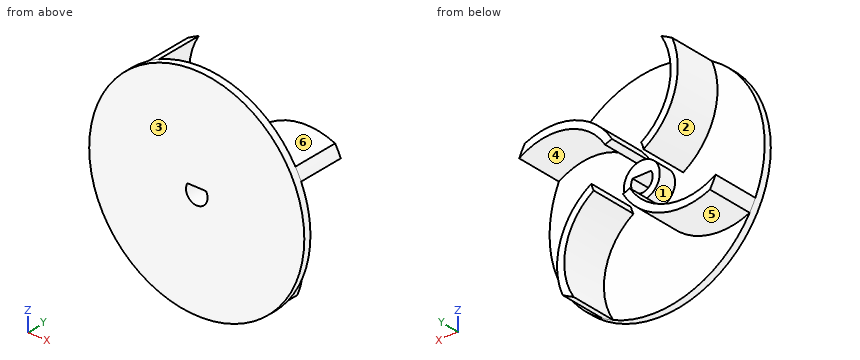
from build123d import *

# Parameters (mm, degrees)
SKETCH1_R           = 30
BOSS_EXTRUDE1_DEPTH = 2
SKETCH2_R           = 5
BOSS_EXTRUDE2_DEPTH = 7
BOSS_EXTRUDE3_DEPTH = 13
CUT_EXTRUDE1_DEPTH  = 16
CIRPATTERN2_COUNT   = 4


with BuildPart() as part:
    # Sketch1 → Boss-Extrude1 (new body)
    with BuildSketch(Plane(origin=(0, 0, 0), x_dir=(1, 0, 0), z_dir=(0, 1, 0))):
        Circle(SKETCH1_R)
    extrude(amount=BOSS_EXTRUDE1_DEPTH)

    # Sketch2 → Boss-Extrude2 (add)
    with BuildSketch(Plane(origin=(0, 0, 0), x_dir=(1, 0, 0), z_dir=(0, 1, 0))):
        Circle(SKETCH2_R)
    extrude(amount=BOSS_EXTRUDE2_DEPTH)

    # Sketch3 → Boss-Extrude3 (add)
    with BuildSketch(Plane(origin=(0, 2, 0), x_dir=(1, 0, 0), z_dir=(0, 1, 0))):
        with BuildLine():
            ThreePointArc((-1.505806951, 7.292266896), (-12.151790035, 15.86929072), (-25.810761164, 15.290670625))
            ThreePointArc((-25.810761164, 15.290670625), (-26.649690738, 13.776573724), (-27.399897799, 12.216611666))
            ThreePointArc((-27.399897799, 12.216611666), (-14.251932533, 14.383859932), (-3.429686075, 6.60922571))
            ThreePointArc((-3.429686075, 6.60922571), (-2.491266579, 7.016993793), (-1.505806951, 7.292266896))
        make_face()
    boss_extrude3 = extrude(amount=BOSS_EXTRUDE3_DEPTH)

    # Sketch4 → Cut-Extrude1 (cut, through all)
    with BuildSketch(Plane(origin=(0, 0, 0), x_dir=(1, 0, 0), z_dir=(0, 1, 0))):
        with BuildLine():
            Line((-2.598076211, -1.5), (2.598076211, -1.5))
            ThreePointArc((2.598076211, -1.5), (0, 3), (-2.598076211, -1.5))
        make_face()
    extrude(amount=CUT_EXTRUDE1_DEPTH, mode=Mode.SUBTRACT)

    # CirPattern2: Boss-Extrude3 ×4 about axis
    cirpattern2_axis = Axis((0, 0, 0), (0, 1, 0))
    for i in range(1, CIRPATTERN2_COUNT):
        add(boss_extrude3.rotate(cirpattern2_axis, i * 360 / CIRPATTERN2_COUNT))


solid = part.part
Here's how the part is built. I have some questions about the finished solid (model axes, mm). Face numbers are marked on the shaded views. A direction names the side the tool comes from. Round coordinates to 2 decimals unless told otherwise and drop trailing zeros. Write each loop counter-clockwise with the first axis right and the second up, starting at its lowest first coordinate (ties: lowest second). Pieces come first, ordered by that corner, then holes.
1. Suppose I cut it at B-B (z = 0). List the corners of the cut face in (x, y) for me.
2. I need wall thicknesses on L1, parallel to Z at x = 0, y = 4.5; L2, parallel to X at y = 3, z = -2.5; L3, parallel to X at y = 2.25, z = 0. Which ranges of each line are inside material? Lowest first, please.
3. Will these pins go through, and if not, where does the flat tip stop? pin 1 Ø5 at (x, z) = (-1, 1) entering from +Y; pin 2 Ø6 at (x, z) = (4.5, -17) entering from +Y; pin 3 Ø5.5 at (x, y) = (-0.5, 2) entering from -Z; pin 4 Ø2 at (y, z) = (8.5, 3.5) entering from +X.
4. Suppose I cut it at A-A (y = 4.5). List the corners of the cut face in (x, z) for me, and give its area (3 significant figures).
5. Suppose I cut it at D-D (y = 13.25). List the corners of the cut face in (x, z) for me.
6. For the marked faces 4, 5 and 6, which set-ups out of +Z, -Z, +X, -X, +Y, -Y let a thin tool reach every point of the face, with its end or its side?
7. Suppose I cut it at C-C (x = 0). List the corners of the cut face in (y, z) for me.
8. If we mould it in two halves opening along X, with no side actions, what happens to the marked faces 1, 2 and 3? For each: released by +X, released by -X, zero draft, split by the parting line, or undercut.
Answer sheet:
1. outline: (-30, 0) - (-3, 0) - (-3, 7) - (-5, 7) - (-5, 2) - (-30, 2) - close; (3, 0) - (30, 0) - (30, 2) - (5, 2) - (5, 7) - (3, 7) - close
2. L1: z = -5 to -3, 1.5 to 5
2. L2: x = -4.33 to -1.66, 1.66 to 4.33, 7.01 to 8.81
2. L3: x = -5 to -3, 3 to 5
3. pin 1: stops at y = 7
3. pin 2: stops at y = 2
3. pin 3: stops at z = -30
3. pin 4: stops at x = -6.61
4. outline: (-27.4, -12.22) arc R30 ccw to (-25.81, -15.29) arc R19.39 ccw to (-1.51, -7.29) arc R7.45 cw to (-3.43, -6.61) arc R17.39 cw to start; (-15.29, 25.81) arc R19.39 ccw to (-7.29, 1.51) arc R7.45 cw to (-6.61, 3.43) arc R17.39 cw to (-12.22, 27.4) arc R30 ccw to start; circle Ø10 at (0, 0); (1.51, 7.29) arc R7.45 cw to (3.43, 6.61) arc R17.39 cw to (27.4, 12.22) arc R30 ccw to (25.81, 15.29) arc R19.39 ccw to start; (6.61, -3.43) arc R17.39 cw to (12.22, -27.4) arc R30 ccw to (15.29, -25.81) arc R19.39 ccw to (7.29, -1.51) arc R7.45 cw to start; hole (-2.6, 1.5) arc R3 ccw (long way) to (2.6, 1.5) - close
4. area: 277 mm2
5. outline: (-27.4, -12.22) arc R30 ccw to (-25.81, -15.29) arc R19.39 ccw to (-1.51, -7.29) arc R7.45 cw to (-3.43, -6.61) arc R17.39 cw to start; (-15.29, 25.81) arc R19.39 ccw to (-7.29, 1.51) arc R7.45 cw to (-6.61, 3.43) arc R17.39 cw to (-12.22, 27.4) arc R30 ccw to start; (1.51, 7.29) arc R7.45 cw to (3.43, 6.61) arc R17.39 cw to (27.4, 12.22) arc R30 ccw to (25.81, 15.29) arc R19.39 ccw to start; (6.61, -3.43) arc R17.39 cw to (12.22, -27.4) arc R30 ccw to (15.29, -25.81) arc R19.39 ccw to (7.29, -1.51) arc R7.45 cw to start
6. face 4: +Y
6. face 5: -Z, +Y
6. face 6: +Z, +Y
7. outline: (0, -30) - (2, -30) - (2, -5) - (7, -5) - (7, -3) - (0, -3) - close; (0, 1.5) - (7, 1.5) - (7, 5) - (2, 5) - (2, 30) - (0, 30) - close
8. face 1: undercut
8. face 2: released by -X
8. face 3: zero draft
